```python
from build123d import *

# Parameters (mm, degrees)
SKETCH1_R           = 90
SKETCH1_R_2         = 64
BOSS_EXTRUDE1_DEPTH = 18
SKETCH2_R           = 90
BOSS_EXTRUDE2_DEPTH = 1
SKETCH3_R           = 90
SKETCH3_R_2         = 74
CUT_EXTRUDE1_DEPTH  = 14
SKETCH4_W           = 10
SKETCH4_H           = 5
SKETCH4_W_2         = 5
SKETCH4_H_2         = 10
BOSS_EXTRUDE3_DEPTH = 2
FILLET1_R           = 2
SKETCH5_R           = 1.75
CUT_EXTRUDE2_DEPTH  = 75


with BuildPart() as part:
    # Sketch1 → Boss-Extrude1 (new body)
    with BuildSketch(Plane(origin=(0, 0, 0), x_dir=(1, 0, 0), z_dir=(0, 1, 0))):
        with Locations(Location((0, 0, 0), (0, 0, 270))):
            Circle(SKETCH1_R)
        with Locations(Location((0, 0, 0), (0, 0, 270))):
            Circle(SKETCH1_R_2, mode=Mode.SUBTRACT)
    extrude(amount=BOSS_EXTRUDE1_DEPTH)

    # Sketch2 → Boss-Extrude2 (add)
    with BuildSketch(Plane(origin=(0, 18, 0), x_dir=(1, 0, 0), z_dir=(0, 1, 0))):
        with Locations(Location((0, 0, 0), (0, 0, 270))):
            Circle(SKETCH2_R)
    extrude(amount=BOSS_EXTRUDE2_DEPTH)

    # Sketch3 → Cut-Extrude1 (cut)
    with BuildSketch(Plane.XZ):
        with Locations(Location((0, 0, 0), (0, 0, 270))):
            Circle(SKETCH3_R)
        with Locations(Location((0, 0, 0), (0, 0, 270))):
            Circle(SKETCH3_R_2, mode=Mode.SUBTRACT)
    extrude(amount=-CUT_EXTRUDE1_DEPTH, mode=Mode.SUBTRACT)

    # Sketch4 → Boss-Extrude3 (add)
    with BuildSketch(Plane.XZ):
        with Locations((0, 64)):
            Rectangle(SKETCH4_W, SKETCH4_H)
        with Locations((-64, 0)):
            Rectangle(SKETCH4_W_2, SKETCH4_H_2)
        with Locations((64, 0)):
            Rectangle(SKETCH4_W_2, SKETCH4_H_2)
        with Locations((0, -64)):
            Rectangle(SKETCH4_W, SKETCH4_H)
    extrude(amount=-BOSS_EXTRUDE3_DEPTH)

    # Fillet1
    # the kernel refuses this fillet: 2 mm, written as the material it takes off along each edge
    with BuildSketch(Plane(origin=(-61.5, 0, 5), x_dir=(-1, 0, 0), z_dir=(0, 0, -1)), Plane(origin=(-5, 2, 61.5), x_dir=(0, 0, 1), z_dir=(1, 0, 0)), Plane(origin=(61.5, 2, 5), x_dir=(1, 0, 0), z_dir=(0, 0, -1)), Plane(origin=(5, 2, -61.5), x_dir=(0, 0, -1), z_dir=(-1, 0, 0))) as fillet1_piece_1:
        with BuildLine():
            CenterArc((FILLET1_R, FILLET1_R), FILLET1_R, 180, 90)
            Line((0, FILLET1_R), (0, 0))
            Line((0, 0), (FILLET1_R, 0))
        make_face()
    extrude(amount=10, mode=Mode.SUBTRACT)
    with BuildSketch(Plane(origin=(-61.5, 2, 5), x_dir=(-1, 0, 0), z_dir=(0, 0, -1)), Plane(origin=(-5, 0, 61.5), x_dir=(0, 0, 1), z_dir=(1, 0, 0)), Plane(origin=(61.5, 0, 5), x_dir=(1, 0, 0), z_dir=(0, 0, -1)), Plane(origin=(5, 0, -61.5), x_dir=(0, 0, -1), z_dir=(-1, 0, 0))) as fillet1_piece_2:
        with BuildLine():
            CenterArc((FILLET1_R, -FILLET1_R), FILLET1_R, 90, 90)
            Line((0, -FILLET1_R), (0, 0))
            Line((0, 0), (FILLET1_R, 0))
        make_face()
    extrude(amount=10, mode=Mode.SUBTRACT)
    with BuildSketch(Plane(origin=(-61.5, -5, 5), x_dir=(-1, 0, 0), z_dir=(0, 1, 0)), Plane(origin=(5, -5, 61.5), x_dir=(0, 0, 1), z_dir=(0, 1, 0)), Plane(origin=(61.5, -5, -5), x_dir=(1, 0, 0), z_dir=(0, 1, 0)), Plane(origin=(-5, -5, -61.5), x_dir=(0, 0, -1), z_dir=(0, 1, 0))) as fillet1_piece_3:
        with BuildLine():
            CenterArc((FILLET1_R, -FILLET1_R), FILLET1_R, 90, 90)
            Line((0, -FILLET1_R), (0, 0))
            Line((0, 0), (FILLET1_R, 0))
        make_face()
    extrude(amount=12, mode=Mode.SUBTRACT)
    with BuildSketch(Plane(origin=(-61.5, -5, -5), x_dir=(-1, 0, 0), z_dir=(0, 1, 0)), Plane(origin=(-5, -5, 61.5), x_dir=(0, 0, 1), z_dir=(0, 1, 0)), Plane(origin=(61.5, -5, 5), x_dir=(1, 0, 0), z_dir=(0, 1, 0)), Plane(origin=(5, -5, -61.5), x_dir=(0, 0, -1), z_dir=(0, 1, 0))) as fillet1_piece_4:
        with BuildLine():
            CenterArc((FILLET1_R, FILLET1_R), FILLET1_R, 180, 90)
            Line((0, FILLET1_R), (0, 0))
            Line((0, 0), (FILLET1_R, 0))
        make_face()
    extrude(amount=12, mode=Mode.SUBTRACT)

    # Sketch5 → Cut-Extrude2 (cut)
    with BuildSketch(Plane.XZ.offset(-14)):
        with Locations(Location((0, 81.969345849, 0), (0, 0, 270))):
            Circle(SKETCH5_R)
        with Locations(Location((81.969345849, 0, 0), (0, 0, 270))):
            Circle(SKETCH5_R)
        with Locations(Location((0, -81.969345849, 0), (0, 0, 270))):
            Circle(SKETCH5_R)
        with Locations(Location((-81.969345849, 0, 0), (0, 0, 270))):
            Circle(SKETCH5_R)
    extrude(amount=-CUT_EXTRUDE2_DEPTH, mode=Mode.SUBTRACT)


solid = part.part
```
Design review of the part built by this model. Coordinates are the model's own, in mm. A direction names the side the tool comes from. Coordinates: 2 decimals unless noted, no trailing zeros. Write each loop counter-clockwise with the first axis right and the second up, starting at its lowest first coordinate (ties: lowest second). Pieces come first, ordered by that corner, then holes.
1) Add section B-B (x = -13). Write out the cut boundary in (y, z).
2) Add section C-C (y = 5.5). Write out the cut boundary in (x, z).
3) Add section D-D (x = -69). Write out the cut boundary in (y, z), plus the area to 3 significant figures.
4) Mouldability with a two-part tool opening along Z and no side actions: class faces 3 (the flat face through (1, 19, -1)), 4 (the cylindrical face through (-24.51, 8.87, 59.12)), 5 (the cylindrical face through (-28.34, 6.9, -68.36)) as +Z half, -Z half, draft (parallel to the pull), parting line (faces both ways), or undercut.
5) Insertion check: pin 1 (2 mm diameter, centred on x = -7.5, z = 44.5, fed in from -Y); pin 2 (4 mm diameter, centred on x = 0, z = 81.97, fed in from -Y); pin 3 (2 mm diameter, centred on y = 17, z = 23.5, fed in from -X); pin 4 (2 mm diameter, centred on x = 81.97, z = 0, fed in from +Y). Each pin has a flat end and moves straight along its axis. Give the tip position at first contact, or say it passes through.
6) To check wall thickness, follow L1, parallel to X at y = 16.35, z = 0; L2, parallel to Y at x = 76, z = -47; L3, parallel to Y at x = 54, z = 8. State the ranges of each line that lie inside material, in increasing order.
7) Add section A-A (z = 25). Write out the cut boundary in (x, y), plus the area to 3 significant figures.
8) Machinability: for faces 1 (the cylindrical face through (-34.471, 16.465, 83.137)), 2 (the flat face through (-66, 14, 34)), which of the approach directions +Z, -Z, +X, -X, +Y, -Y give a long, thin tool a straight path to every point of the face, cutting with its end or side? Answer none if there is none.
Check result:
1. outline: (0, -72.85) - (14, -72.85) - (14, -89.06) - (19, -89.06) - (19, 89.06) - (14, 89.06) - (14, 72.85) - (0, 72.85) - (0, 62.67) - (18, 62.67) - (18, -62.67) - (0, -62.67) - close
2. outline: circle Ø148 at (0, 0); hole circle Ø128 at (0, 0)
3. outline: (0, -26.74) - (14, -26.74) - (14, -57.78) - (19, -57.78) - (19, 57.78) - (14, 57.78) - (14, 26.74) - (0, 26.74) - close
3. area: 1,330 mm2
4. face 3: draft
4. face 4: undercut
4. face 5: parting line
5. pin 1: stops at y = 18
5. pin 2: stops at y = 14
5. pin 3: stops at x = -87.14
5. pin 4: passes through
6. L1: x = -90 to -83.72, -80.22 to -64, 64 to 80.22, 83.72 to 90
6. L2: y = 14 to 19
6. L3: y = 18 to 19
7. outline: (-86.46, 14) - (-69.65, 14) - (-69.65, 0) - (-58.92, 0) - (-58.92, 18) - (58.92, 18) - (58.92, 0) - (69.65, 0) - (69.65, 14) - (86.46, 14) - (86.46, 19) - (-86.46, 19) - close
7. area: 694 mm2
8. face 1: +Y, -Y
8. face 2: -Y
